```python
from build123d import *

# Parameters (mm, degrees)
MODEL_R             = 3
MODEL_R_2           = 4.125
BOSS_EXTRUDE1_DEPTH = 10


with BuildPart() as part:
    # Model → Boss-Extrude1 (new body)
    with BuildSketch(Plane.XY):
        with BuildLine():
            Line((36, -25), (-36, -25))
            ThreePointArc((-36, -25), (-38.828427125, -23.828427125), (-40, -21))
            Line((-40, -21), (-40, 21))
            ThreePointArc((-40, 21), (-38.828427125, 23.828427125), (-36, 25))
            Line((-36, 25), (36, 25))
            ThreePointArc((36, 25), (38.828427125, 23.828427125), (40, 21))
            Line((40, 21), (40, -21))
            ThreePointArc((40, -21), (38.828427125, -23.828427125), (36, -25))
        make_face()
        with Locations((32, 17)):
            Circle(MODEL_R, mode=Mode.SUBTRACT)
        with Locations((-32, 17)):
            Circle(MODEL_R, mode=Mode.SUBTRACT)
        with Locations((32, -17)):
            Circle(MODEL_R, mode=Mode.SUBTRACT)
        Circle(MODEL_R_2, mode=Mode.SUBTRACT)
        with Locations((-32, -17)):
            Circle(MODEL_R, mode=Mode.SUBTRACT)
    extrude(amount=BOSS_EXTRUDE1_DEPTH)


solid = part.part
```
Input: part model. Units: mm. Frame: model coordinates. Give positions to 0.01 mm unless a question says otherwise; leave off trailing zeros. Order: outer loops, then holes, each group sorted by start corner. A loop starts at its lowest first (then second) coordinate and runs counter-clockwise, first axis right, second up. Notation, with made-up numbers: (8, 6.25) - (36, 6.25) arc R4 cw to (36, 11.25) - close; hole circle Ø6 at (52.5, 34). An arc over 180 degrees is marked (long way). Put each result on its own line as item: value.
Item 1: Section query B-B, the plane x = 32. Return loops of the section in (y, z).
Found:
outline: (-25, 0) - (-20, 0) - (-20, 10) - (-25, 10) - close; (-14, 0) - (14, 0) - (14, 10) - (-14, 10) - close; (20, 0) - (25, 0) - (25, 10) - (20, 10) - close
Item 2: Draft query along Y for faces 1 (the cylindrical face through (38.797, 23.859, 4.93)), 2 (the flat face through (-40, 0, 5)), 3 (the cylindrical face through (-35, 17, 5)), 4 (the cylindrical face through (-35, -17, 5)). Return one class per face: +Y half, -Y half, draft (parallel to the pull), parting line (faces both ways), or undercut.
Found:
face 1: +Y half
face 2: draft
face 3: undercut
face 4: undercut
Item 3: Section query D-D, the plane z = 3.75. Return loops of the section in (x, y) (3 decimals), then the cut area to 3 significant figures.
Found:
outline: (-40, -21) arc R4 ccw to (-36, -25) - (36, -25) arc R4 ccw to (40, -21) - (40, 21) arc R4 ccw to (36, 25) - (-36, 25) arc R4 ccw to (-40, 21) - close; hole circle Ø6 at (-32, -17); hole circle Ø6 at (-32, 17); hole circle Ø8.25 at (0, 0); hole circle Ø6 at (32, -17); hole circle Ø6 at (32, 17)
area: 3,820 mm^2
Item 4: Ray query, L1, parallel to Y at x = 32, z = 2; L2, parallel to Y at x = 31, z = 8.5; L3, parallel to Y at x = 0, z = 2.25 (3 decimals). Return the intervals inside material, ascending. Write a range as from..to.
Found:
L1: y = -25..-20, -14..14, 20..25
L2: y = -25..-19.83, -14.17..14.17, 19.83..25
L3: y = -25..-4.125, 4.125..25
Item 5: Contact query for a flat-ended pin moving along its axis: pin 1 (4 mm diameter, centred on x = 18.5, y = -10.5, fed in from -Z). Output: stop coordinate, or through.
Found:
pin 1: stops at z = 0
Item 6: Section query C-C, the plane y = -17. Return loops of the section in (x, z), then the cut area to 3 significant figures.
Found:
outline: (-40, 0) - (-35, 0) - (-35, 10) - (-40, 10) - close; (-29, 0) - (29, 0) - (29, 10) - (-29, 10) - close; (35, 0) - (40, 0) - (40, 10) - (35, 10) - close
area: 680 mm^2
Item 7: Section query A-A, the plane y = 0. Return loops of the section in (x, z) (3 decimals), then the cut area to 4 significant figures.
Found:
outline: (-40, 0) - (-4.125, 0) - (-4.125, 10) - (-40, 10) - close; (4.125, 0) - (40, 0) - (40, 10) - (4.125, 10) - close
area: 717.5 mm^2
